Could you check a few things on this drawing? It's one solid part, dimensions in mm from its lowest x, y, z. A direction names the side the tool comes from. Give positions to 0.01 mm unless a question says otherwise; leave off trailing zeros. Write each loop counter-clockwise with the first axis right and the second up, starting at its lowest first coordinate (ties: lowest second). Pieces come first, ordered by that corner, then holes. Notation, with made-up numbers: M -19,88.25 L 36,88.25 A26 cw 36,125.25 Z; hole C -2,13.25 d3. An arc over 180 degrees is marked long. Write each question's results on one line, items separated by ' | '. Start each with the question number.
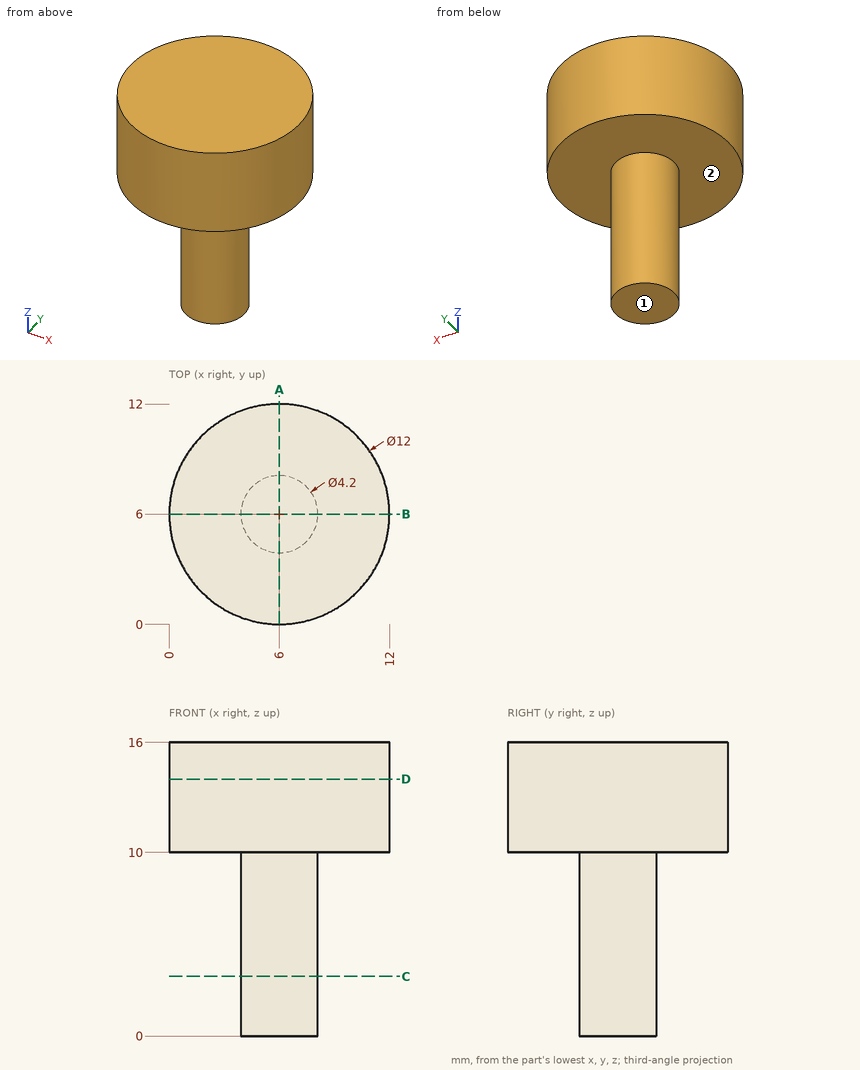
Q1. If we section it at A-A (x = 6): Please give me the cut outline in (y, z).
Q2. I'm going to push flat-ended pins straight in: P1, Ø1, axis at y = 6.5, z = 6, coming from the -X side; P2, Ø1, axis at x = 4.5, z = 13.5, coming from the +Y side. Where does each tip first touch, or does it pass through?
Q3. If we section it at C-C (z = 3.25): Please give me the cut outline in (x, y), plus the area to 3 significant figures.
Q4. If we section it at D-D (z = 14): Please give me the cut outline in (x, y), plus the area to 3 significant figures.
Q5. Please list where these lines run through material, in increasing order: line 1 (Z direction, x = 4.75, y = 1.75); line 2 (X direction, y = 6.25, z = 4); line 3 (X direction, y = 4.25, z = 2.5). Write a range as [from, to].
Q6. For the marked faces 1 and 2, which set-ups out of +Z, -Z, +X, -X, +Y, -Y let a thin tool reach every point of the face, with its end or its side?
Determined:
1) outline: M 0,10 L 3.9,10 L 3.9,0 L 8.1,0 L 8.1,10 L 12,10 L 12,16 L 0,16 Z
2) P1: stops at x = 3.9 | P2: stops at y = 11.92
3) outline: C 6,6 d4.2 | area: 13.9 mm²
4) outline: C 6,6 d12 | area: 113 mm²
5) line 1: z = [10, 16] | line 2: x = [3.91, 8.09] | line 3: x = [4.84, 7.16]
6) face 1: -Z, +X, -X, +Y, -Y | face 2: -Z
